The model under review builds one solid part; all positions refer to its coordinate system, in mm. Coordinates: 2 decimals unless noted, no trailing zeros. Write each loop counter-clockwise with the first axis right and the second up, starting at its lowest first coordinate (ties: lowest second). Pieces come first, ordered by that corner, then holes.
1) Add section B-B, the plane y = 1.1. State the section outline as (x, z) points (3 decimals), then the cut area to 3 significant figures.
2) For line 1 (Z direction, x = 71.2, y = 0.8); line 2 (Z direction, x = 8.5, y = 0.9) (3 decimals); line 3 (Z direction, x = -54, y = 1.3), list the stretches that pass through material, from the lowest coordinate up.
3) Add section A-A, the plane z = 20. State the section outline as (x, y) points (3 decimals).
4) Add section C-C, the plane x = 71.2. State the section outline as (y, z) points (3 decimals).
5) Add section D-D, the plane x = -20.5. State the section outline as (y, z) points (3 decimals), then the cut area to 3 significant figures.
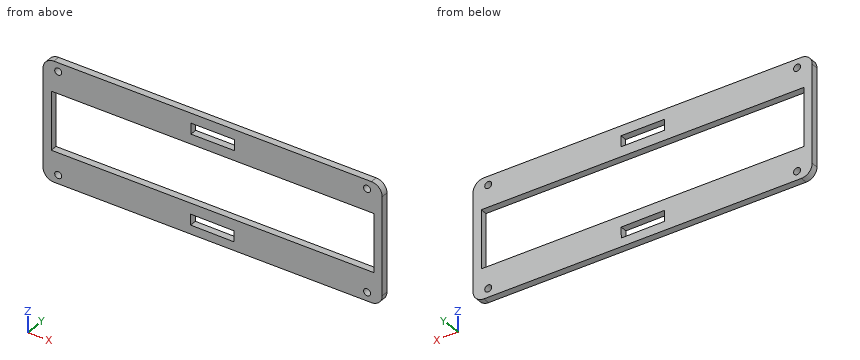
from build123d import *

# Parameters (mm, degrees)
SKETCH2_W           = 156.4
SKETCH2_H           = 55
BOSS_EXTRUDE1_DEPTH = 3.175
SKETCH3_W           = 148.78
SKETCH3_H           = 26.86
CUT_EXTRUDE1_DEPTH  = 83.955232656
SKETCH4_R           = 1.6
CUT_EXTRUDE2_DEPTH  = 83.955232656
SKETCH5_W           = 20
SKETCH5_H           = 5
CUT_EXTRUDE3_DEPTH  = 83.955232656
FILLET1_R           = 5
FILLET2_R           = 5


with BuildPart() as part:
    # Sketch2 → Boss-Extrude1 (new body)
    with BuildSketch(Plane(origin=(0, 0, 0), x_dir=(1, 0, 0), z_dir=(0, 1, 0))):
        Rectangle(SKETCH2_W, SKETCH2_H)
    extrude(amount=BOSS_EXTRUDE1_DEPTH)

    # Sketch3 → Cut-Extrude1 (cut, through all)
    with BuildSketch(Plane.XZ):
        Rectangle(SKETCH3_W, SKETCH3_H)
    extrude(amount=-CUT_EXTRUDE1_DEPTH, mode=Mode.SUBTRACT)

    # Sketch4 → Cut-Extrude2 (cut, through all)
    with BuildSketch(Plane(origin=(0, 3.175, 0), x_dir=(1, 0, 0), z_dir=(0, 1, 0))):
        with Locations(Location((-71.2, -23.5, 0), (0, 0, 270))):
            Circle(SKETCH4_R)
        with Locations(Location((-71.2, 23.5, 0), (0, 0, 90))):
            Circle(SKETCH4_R)
        with Locations(Location((71.2, 23.5, 0), (0, 0, 270))):
            Circle(SKETCH4_R)
        with Locations(Location((71.2, -23.5, 0), (0, 0, 90))):
            Circle(SKETCH4_R)
    extrude(amount=-CUT_EXTRUDE2_DEPTH, mode=Mode.SUBTRACT)

    # Sketch5 → Cut-Extrude3 (cut, through all)
    with BuildSketch(Plane(origin=(0, 3.175, 0), x_dir=(1, 0, 0), z_dir=(0, 1, 0))):
        with Locations((0, -20.465)):
            Rectangle(SKETCH5_W, SKETCH5_H)
        Polygon((-10.154798185, 23.41968691), (-10.121425865, 18.419798282), (9.878128645, 18.553287562), (9.844756325, 23.553176189), align=None)
    extrude(amount=-CUT_EXTRUDE3_DEPTH, mode=Mode.SUBTRACT)

    # Fillet1
    fillet1_edges = [part.edges().sort_by_distance(p)[0] for p in [
        (78.2, 1.5875, 27.5),
        (-78.2, 1.5875, 27.5),
        (-78.2, 1.5875, -27.5),
    ]]
    fillet(fillet1_edges, radius=FILLET1_R)

    # Fillet2
    fillet2_edges = [part.edges().sort_by_distance(p)[0] for p in [
        (78.2, 1.5875, -27.5),
    ]]
    fillet(fillet2_edges, radius=FILLET2_R)


solid = part.part
Geometry results:
1. outline: (-78.2, -22.5) arc R5 ccw to (-73.2, -27.5) - (73.2, -27.5) arc R5 ccw to (78.2, -22.5) - (78.2, 22.5) arc R5 ccw to (73.2, 27.5) - (-73.2, 27.5) arc R5 ccw to (-78.2, 22.5) - close; hole (-74.39, -13.43) - (74.39, -13.43) - (74.39, 13.43) - (-74.39, 13.43) - close; hole circle Ø3.2 at (-71.2, -23.5); hole circle Ø3.2 at (-71.2, 23.5); hole (-10.155, -23.42) - (9.845, -23.553) - (9.878, -18.553) - (-10.121, -18.42) - close; hole (-10, 17.965) - (10, 17.965) - (10, 22.965) - (-10, 22.965) - close; hole circle Ø3.2 at (71.2, -23.5); hole circle Ø3.2 at (71.2, 23.5)
1. area: 4,350 mm2
2. line 1: z = -27.5 to -25.1, -21.9 to -13.43, 13.43 to 21.9, 25.1 to 27.5
2. line 2: z = -27.5 to -23.544, -18.544 to -13.43, 13.43 to 17.965, 22.965 to 27.5
2. line 3: z = -27.5 to -13.43, 13.43 to 27.5
3. outline: (-78.2, 0) - (-10, 0) - (-10, 3.175) - (-78.2, 3.175) - close; (10, 0) - (78.2, 0) - (78.2, 3.175) - (10, 3.175) - close
4. outline: (0, -27.5) - (3.175, -27.5) - (3.175, -25.1) - (0, -25.1) - close; (0, -21.9) - (3.175, -21.9) - (3.175, -13.43) - (0, -13.43) - close; (0, 13.43) - (3.175, 13.43) - (3.175, 21.9) - (0, 21.9) - close; (0, 25.1) - (3.175, 25.1) - (3.175, 27.5) - (0, 27.5) - close
5. outline: (0, -27.5) - (3.175, -27.5) - (3.175, -13.43) - (0, -13.43) - close; (0, 13.43) - (3.175, 13.43) - (3.175, 27.5) - (0, 27.5) - close
5. area: 89.3 mm2
